Geometry: final body of the model. Coordinates: model frame, mm. A direction names the side the tool comes from. Give positions to 0.01 mm unless a question says otherwise; leave off trailing zeros. Loops run counter-clockwise (first coordinate to the right, second up) from the corner with the lowest first, then second, coordinate; pieces in that order, holes last.
1. First-contact query: P1, Ø8, axis at x = -18.5, z = 12, coming from the -Y side; P2, Ø3, axis at x = -5, y = -36, coming from the -Z side; P3, Ø5, axis at x = -8.5, y = -37, coming from the -Z side. Flat tips, straight axial feed; report the tip coordinate or a pass-through.
2. Material intervals for line 1 along Y through (x, z) = (20, 6.5); line 2 along X through (y, z) = (-40.5, 1); line 3 along X through (y, z) = (-40, 17.25), sorted ascending.
3. Section B-B, the plane z = 10. Output: boundary loops of the cut face in (x, y).
4. Section A-A, the plane x = 20. Output: boundary loops of the cut face in (y, z).
5. Section C-C, the plane y = -43.75. Output: boundary loops of the cut face in (x, z), then the cut area to 3 significant figures.
6. Access query for faces 5 (the face through (12, -41, 0)), 6 (the face through (-12.3, -44.6, 10.5)). Directions: +Z, -Z, +X, -X, +Y, -Y. A direction counts if a zero-diameter tool reaches every point of the face in a straight line with its end or side. Return the directions, or none.
7. Section D-D, the plane z = 4.5. Output: boundary loops of the cut face in (x, y), then the cut area to 3 significant figures.
8. Draft query along X for faces 1 (the face through (25, -41, 10)), 2 (the face through (0, -40.5, 5.7)), 3 (the face through (12, -34.631, 10)), 4 (the face through (18.016, -42.152, 10.14)). Return one class per face: +X half, -X half, draft (parallel to the pull), parting line (faces both ways), or undercut.
from build123d import *

# Parameters (mm, degrees)
SKETCH_1_W          = 20
SKETCH_1_H          = 12
EXTRUDE_1_DEPTH     = 25
SKETCH_5_R          = 2.5
CUT_EXTRUDE_2_DEPTH = 57.563315968
SKETCH1_R           = 4
BOSS_EXTRUDE1_DEPTH = 25


with BuildPart() as part:
    # Эскиз1 → Вытянуть1 (new body)
    with BuildSketch(Plane(origin=(0, 0, 0), x_dir=(0, 0, -1), z_dir=(1, 0, 0))):
        with Locations((-10, -40.630555576)):
            Rectangle(SKETCH_1_W, SKETCH_1_H)
    extrude(amount=EXTRUDE_1_DEPTH)

    # Эскиз5 → Вырез-Вытянуть2 (cut, through all)
    with BuildSketch(Plane.XY.offset(20)):
        with Locations((20, -40.630555576)):
            Circle(SKETCH_5_R)
    extrude(amount=-CUT_EXTRUDE_2_DEPTH, mode=Mode.SUBTRACT)

    # Sketch1 → Boss-Extrude1 (add)
    with BuildSketch(Plane.ZY):
        with Locations(Location((10, -40.630555576, 0), (0, 0, 180))):
            Circle(SKETCH1_R)
    extrude(amount=BOSS_EXTRUDE1_DEPTH)


solid = part.part
Answers below:
1. P1: stops at y = -44.63
1. P2: stops at z = 7.51
1. P3: stops at z = 6.16
2. line 1: y = -46.63 to -43.13, -38.13 to -34.63
2. line 2: x = 0 to 17.5, 22.5 to 25
2. line 3: x = 0 to 17.58, 22.42 to 25
3. outline: (-25, -44.63) - (0, -44.63) - (0, -46.63) - (25, -46.63) - (25, -34.63) - (0, -34.63) - (0, -36.63) - (-25, -36.63) - close; hole circle Ø5 at (20, -40.63)
4. outline: (-46.63, 0) - (-43.13, 0) - (-43.13, 20) - (-46.63, 20) - close; (-38.13, 0) - (-34.63, 0) - (-34.63, 20) - (-38.13, 20) - close
5. outline: (-25, 7.5) - (0, 7.5) - (0, 0) - (25, 0) - (25, 20) - (0, 20) - (0, 12.5) - (-25, 12.5) - close
5. area: 625 mm2
6. face 5: -Z, +X, -X, +Y, -Y
6. face 6: -X
7. outline: (0, -46.63) - (25, -46.63) - (25, -34.63) - (0, -34.63) - close; hole circle Ø5 at (20, -40.63)
7. area: 280 mm2
8. face 1: +X half
8. face 2: -X half
8. face 3: draft
8. face 4: undercut
